```python
from build123d import *

# Parameters (mm, degrees)
BOX_W     = 40
BOX_H     = 40
BOX_DEPTH = 3
FILLET_R  = 4


with BuildPart() as con001:
    # Cone001 → Cone001 (revolve)
    with BuildSketch(Plane(origin=(20, 20, -0.5), x_dir=(1, 0, 0), z_dir=(0, -1, 0))):
        Polygon((0, 0), (13, 0), (3, 41), (0, 41), align=None)
    revolve(axis=Axis((20, 20, -0.5), (0, 0, 1)))


with BuildPart() as cut:
    # Cone → Cone (revolve)
    with BuildSketch(Plane(origin=(20, 20, 0), x_dir=(1, 0, 0), z_dir=(0, -1, 0))):
        Polygon((0, 0), (14, 0), (4, 40), (0, 40), align=None)
    revolve(axis=Axis((20, 20, 0), (0, 0, 1)))

    # Cut: cut Con001
    add(con001.part, mode=Mode.SUBTRACT)


with BuildPart() as fusion:
    # Box → Box (new body)
    with BuildSketch(Plane.XY):
        with Locations((20, 20)):
            Rectangle(BOX_W, BOX_H)
    extrude(amount=BOX_DEPTH)

    # Fillet
    fillet_edges = [fusion.edges().sort_by_distance(p)[0] for p in [
        (0, 0, 1.5),
        (0, 40, 1.5),
        (40, 0, 1.5),
        (40, 40, 1.5),
    ]]
    fillet(fillet_edges, radius=FILLET_R)

    # Fusion: union Cut
    add(cut.part)


solid = fusion.part
```
Here's how the part is built. I have some questions about the finished solid (model axes, mm). A direction names the side the tool comes from. Give positions to 0.01 mm unless a question says otherwise; leave off trailing zeros. Loops run counter-clockwise (first coordinate to the right, second up) from the corner with the lowest first, then second, coordinate; pieces in that order, holes last. Notation, with made-up numbers: (9, 81.5) -> (46, 81.5) arc R13 cw to (46, 86.5) -> close; hole circle Ø5 at (30.5, 87). An arc over 180 degrees is marked (long way). Use one line per item in the form item = value. Start each with the question number.
1) Thinking about a two-plate mould opening in Z: for faces 4 (the face through (26.994, 17.1, 21.759)), 5 (the face through (28.165, 22.571, 21.759)), 6 (the face through (20, 20, 0)), 7 (the face through (20, 0, 1)), which applies, +Z half, -Z half, draft (parallel to the pull), parting line (faces both ways), or undercut?
2) Imagine slicing it at D-D (y = 34.5). Please give me the cut outline in (x, z).
3) Please list where these lines run through material, in increasing order: line 1 along Z through (x, y) = (30.5, 8); line 2 along X through (y, z) = (17, 17); line 3 along X through (y, z) = (16, 17).
4) Which directions (+Z, -Z, +X, -X, +Y, -Y) give clear straight access to the entire face, cutting with the end or side of a thin tool? Please do faces 1 (the face through (6, 20, 3)), 2 (the face through (1.141, 38.797, 1.521)), 3 (the face through (20, 20, 3)).
5) Imagine slicing it at A-A (x = 20). Please give me the cut outline in (y, z).
6) Imagine slicing it at C-C (z = 15). Please give me the cut outline in (x, y), then the cut area to 3 significant figures.
7) For P1, Ø8, axis at y = 11.5, z = 17, coming from the +X side; P2, Ø8, axis at y = 28, z = 11, coming from the -X side; P3, Ø4, axis at y = 26, z = 7, coming from the -X side; P4, Ø3, axis at x = 30.5, z = 27, coming from the -Y side, each with a flat end and sliding along its axis, tell me the tip position at first contact or that it passes through.
Check values:
q1.face_4 = undercut
q1.face_5 = +Z half
q1.face_6 = -Z half
q1.face_7 = draft
q2.outline = (0, 0) -> (40, 0) -> (40, 3) -> (0, 3) -> close
q3.line_1 = 0 to 3
q3.line_2 = 10.72 to 11.8, 28.2 to 29.28
q3.line_3 = 11.11 to 12.24, 27.76 to 28.89
q4.face_1 = +Z
q4.face_2 = +Z, -Z, -X, +Y
q4.face_3 = none
q5.outline = (0, 0) -> (40, 0) -> (40, 3) -> (33.25, 3) -> (24, 40) -> (23.12, 40) -> (32.15, 3) -> (7.85, 3) -> (16.88, 40) -> (16, 40) -> (6.75, 3) -> (0, 3) -> close
q6.outline = circle Ø20.5 at (20, 20); hole circle Ø18.44 at (20, 20)
q6.area = 63.0 mm^2
q7.P1 = 28.93
q7.P2 = 9.16
q7.P3 = 8.25
q7.P4 = through
